Model file for the job. Use its own axes, mm. A direction names the side the tool comes from. Round coordinates to 2 decimals unless told otherwise and drop trailing zeros. Order: outer loops, then holes, each group sorted by start corner. A loop starts at its lowest first (then second) coordinate and runs counter-clockwise, first axis right, second up. Notation, with made-up numbers: (-29.5, 17.5) - (23.5, 17.5) arc R25 ccw to (23.5, 52.5) - close; hole circle Ø5 at (5.25, -7). An arc over 180 degrees is marked (long way). Put each result on its own line as item: value. Start each with the question number.
Item 1: Probe probe 1 along Y at (x, z) = (2.5, 1.35); probe 2 along Y at (x, z) = (5.75, 0.8); probe 3 along X at (y, z) = (1, 0.8). List the from-to ranges inside material, lowest first.
Item 2: Saw through at A-A on x = 6.75. List the corners of the cut face in (y, z), plus the area to 3 significant figures.
Item 3: Which spindle directions (+Z, -Z, +X, -X, +Y, -Y) get a long thin tool onto all of the face, cutting with end or side? Do faces 4 (the face through (0.89, 2.04, 0)), 5 (the face through (-0.822, -3, 1)). Say none if no direction does.
Item 4: Saw through at B-B on y = 10.5. List the corners of the cut face in (x, z).
Item 5: Saw through at C-C on z = 1.15. List the corners of the cut face in (x, y).
Item 6: Saw through at D-D on x = 5.25. State how many separate pieces and enclosed holes the cut face has, plus the area to 3 significant figures.
Item 7: Mould opens along Y. For faces 1 (the face through (3.7, -14.195, 1.1)), 2 (the face through (3, -15.195, 1)), 3 (the face through (-1, 2, 1.4)) say: pulls with the +Y half, pulls with the -Y half, needs draft (parallel to the pull), parting line crosses it, or undercut.
```python
from build123d import *

# Parameters (mm, degrees)
SKETCH_1_W           = 10
SKETCH_1_H           = 34
EXTRUDE_2_DEPTH      = 1.4
SKETCH_2_W           = 8
SKETCH_2_H           = 32
CUT_EXTRUDE_1_DEPTH  = 1.2
SKETCH_4_W           = 1.2
SKETCH_4_H           = 1
CUT_EXTRUDE_4_DEPTH  = 1.2
FILLET_1_R           = 0.5
FILLET_2_R           = 0.5
SKETCH_6_W           = 6.011424245
SKETCH_6_H           = 0.514664245
CUT_EXTRUDE_6_DEPTH  = 0.5
SKETCH_7_W           = 0.498386998
SKETCH_7_H           = 14.972688723
CUT_EXTRUDE_7_DEPTH  = 0.5
SKETCH_8_W           = 0.497690278
SKETCH_8_H           = 27.903913782
CUT_EXTRUDE_8_DEPTH  = 0.5
SKETCH_10_W          = 5.67106867
SKETCH_10_H          = 0.515598409
CUT_EXTRUDE_9_DEPTH  = 0.5
CUT_EXTRUDE_11_REACH = 22.554


with BuildPart() as part:
    # 草图1 → 凸台-拉伸2 (new body)
    with BuildSketch(Plane.XY):
        with Locations((3.178294574, 1.80536099)):
            Rectangle(SKETCH_1_W, SKETCH_1_H)
    extrude(amount=EXTRUDE_2_DEPTH)

    # 草图2 → 切除-拉伸1 (cut)
    with BuildSketch(Plane.XY.offset(1.4)):
        with Locations((3.178294574, 1.80536099)):
            Rectangle(SKETCH_2_W, SKETCH_2_H)
    extrude(amount=-CUT_EXTRUDE_1_DEPTH, mode=Mode.SUBTRACT)

    # 草图4 → 切除-拉伸4 (cut)
    with BuildSketch(Plane.XY.offset(1.4)):
        with Locations((-0.221705426, -14.69463901)):
            Rectangle(SKETCH_4_W, SKETCH_4_H)
    extrude(amount=-CUT_EXTRUDE_4_DEPTH, mode=Mode.SUBTRACT)

    # 圆角1
    fillet_1_edges = [part.edges().sort_by_distance(p)[0] for p in [
        (-1.821705426, -15.19463901, 0.7),
    ]]
    fillet(fillet_1_edges, radius=FILLET_1_R)

    # 圆角2
    fillet_2_edges = [part.edges().sort_by_distance(p)[0] for p in [
        (-1.821705426, 18.80536099, 0.7),
        (8.178294574, 18.80536099, 0.7),
        (8.178294574, -15.19463901, 0.7),
    ]]
    fillet(fillet_2_edges, radius=FILLET_2_R)

    # 草图6 → 切除-拉伸6 (cut)
    with BuildSketch(Plane.XZ.offset(-17.80536099)):
        with Locations((3.184006697, 0.642667877)):
            Rectangle(SKETCH_6_W, SKETCH_6_H)
    extrude(amount=-CUT_EXTRUDE_6_DEPTH, mode=Mode.SUBTRACT)

    # 草图7 → 切除-拉伸7 (cut)
    with BuildSketch(Plane(origin=(-0.821705426, 0, 0), x_dir=(0, 0, -1), z_dir=(1, 0, 0))):
        with Locations((-0.650806501, 8.293480481)):
            Rectangle(SKETCH_7_W, SKETCH_7_H)
    extrude(amount=-CUT_EXTRUDE_7_DEPTH, mode=Mode.SUBTRACT)

    # 草图8 → 切除-拉伸8 (cut)
    with BuildSketch(Plane.ZY.offset(-7.178294574)):
        with Locations((0.641533001, 1.822842427)):
            Rectangle(SKETCH_8_W, SKETCH_8_H)
    extrude(amount=-CUT_EXTRUDE_8_DEPTH, mode=Mode.SUBTRACT)

    # 草图10 → 切除-拉伸9 (cut)
    with BuildSketch(Plane(origin=(0, -14.19463901, 0), x_dir=(1, 0, 0), z_dir=(0, 1, 0))):
        with Locations((3.213828909, -0.642200795)):
            Rectangle(SKETCH_10_W, SKETCH_10_H)
    extrude(amount=-CUT_EXTRUDE_9_DEPTH, mode=Mode.SUBTRACT)

    # 草图11 → 切除-拉伸11 (cut, up to next)
    with BuildSketch(Plane(origin=(0, 0, 0), x_dir=(-1, 0, 0), z_dir=(0, 0, -1)), mode=Mode.PRIVATE) as cut_extrude_11_sk1:
        with BuildLine():
            Line((-4.31947378, 17.019101686), (-0.131341084, 13.086732818))
            ThreePointArc((-0.131341084, 13.086732818), (-0.078041772, 11.394479644), (-1.770294947, 11.341180331))
            Line((-1.770294947, 11.341180331), (-5.958427643, 15.273549198))
            ThreePointArc((-5.958427643, 15.273549198), (-6.011726955, 16.965802373), (-4.31947378, 17.019101686))
        make_face()
    cut_extrude_11_tool1 = extrude(cut_extrude_11_sk1.sketch, amount=-CUT_EXTRUDE_11_REACH, mode=Mode.PRIVATE) & part.part
    # 草图11 → 切除-拉伸11 (cut, up to next)
    with BuildSketch(Plane(origin=(0, 0, 0), x_dir=(-1, 0, 0), z_dir=(0, 0, -1)), mode=Mode.PRIVATE) as cut_extrude_11_sk2:
        with BuildLine():
            Line((-5.958427643, 9.273549198), (-1.770294947, 5.341180331))
            ThreePointArc((-1.770294947, 5.341180331), (-0.078041772, 5.394479644), (-0.131341084, 7.086732818))
            Line((-0.131341084, 7.086732818), (-4.31947378, 11.019101686))
            ThreePointArc((-4.31947378, 11.019101686), (-6.011726955, 10.965802373), (-5.958427643, 9.273549198))
        make_face()
    cut_extrude_11_tool2 = extrude(cut_extrude_11_sk2.sketch, amount=-CUT_EXTRUDE_11_REACH, mode=Mode.PRIVATE) & part.part
    # 草图11 → 切除-拉伸11 (cut, up to next)
    with BuildSketch(Plane(origin=(0, 0, 0), x_dir=(-1, 0, 0), z_dir=(0, 0, -1)), mode=Mode.PRIVATE) as cut_extrude_11_sk3:
        with BuildLine():
            Line((-5.958427643, 3.273549198), (-1.770294947, -0.658819669))
            ThreePointArc((-1.770294947, -0.658819669), (-0.078041772, -0.605520356), (-0.131341084, 1.086732818))
            Line((-0.131341084, 1.086732818), (-4.31947378, 5.019101686))
            ThreePointArc((-4.31947378, 5.019101686), (-6.011726955, 4.965802373), (-5.958427643, 3.273549198))
        make_face()
    cut_extrude_11_tool3 = extrude(cut_extrude_11_sk3.sketch, amount=-CUT_EXTRUDE_11_REACH, mode=Mode.PRIVATE) & part.part
    # 草图11 → 切除-拉伸11 (cut, up to next)
    with BuildSketch(Plane(origin=(0, 0, 0), x_dir=(-1, 0, 0), z_dir=(0, 0, -1)), mode=Mode.PRIVATE) as cut_extrude_11_sk4:
        with BuildLine():
            Line((-5.958427643, -2.726450802), (-1.770294947, -6.658819669))
            ThreePointArc((-1.770294947, -6.658819669), (-0.078041772, -6.605520356), (-0.131341084, -4.913267182))
            Line((-0.131341084, -4.913267182), (-4.31947378, -0.980898314))
            ThreePointArc((-4.31947378, -0.980898314), (-6.011726955, -1.034197627), (-5.958427643, -2.726450802))
        make_face()
    cut_extrude_11_tool4 = extrude(cut_extrude_11_sk4.sketch, amount=-CUT_EXTRUDE_11_REACH, mode=Mode.PRIVATE) & part.part
    # 草图11 → 切除-拉伸11 (cut, up to next)
    with BuildSketch(Plane(origin=(0, 0, 0), x_dir=(-1, 0, 0), z_dir=(0, 0, -1)), mode=Mode.PRIVATE) as cut_extrude_11_sk5:
        with BuildLine():
            Line((-5.958427643, -8.726450802), (-1.770294947, -12.658819669))
            ThreePointArc((-1.770294947, -12.658819669), (-0.078041772, -12.605520356), (-0.131341084, -10.913267182))
            Line((-0.131341084, -10.913267182), (-4.31947378, -6.980898314))
            ThreePointArc((-4.31947378, -6.980898314), (-6.011726955, -7.034197627), (-5.958427643, -8.726450802))
        make_face()
    cut_extrude_11_tool5 = extrude(cut_extrude_11_sk5.sketch, amount=-CUT_EXTRUDE_11_REACH, mode=Mode.PRIVATE) & part.part
    add(cut_extrude_11_tool1.solids().sort_by_distance((3.044884, 14.180141, 0))[0], mode=Mode.SUBTRACT)
    add(cut_extrude_11_tool2.solids().sort_by_distance((3.044884, 8.180141, 0))[0], mode=Mode.SUBTRACT)
    add(cut_extrude_11_tool3.solids().sort_by_distance((3.044884, 2.180141, 0))[0], mode=Mode.SUBTRACT)
    add(cut_extrude_11_tool4.solids().sort_by_distance((3.044884, -3.819859, 0))[0], mode=Mode.SUBTRACT)
    add(cut_extrude_11_tool5.solids().sort_by_distance((3.044884, -9.819859, 0))[0], mode=Mode.SUBTRACT)


solid = part.part
```
Results found:
1. probe 1: y = -15.19 to -14.19, 17.81 to 18.81
1. probe 2: y = -15.19 to -14.69, 18.31 to 18.81
1. probe 3: x = -1.82 to -1.32, 7.68 to 8.18
2. outline: (-15.19, 0) - (18.81, 0) - (18.81, 1.4) - (17.81, 1.4) - (17.81, 0.2) - (-14.19, 0.2) - (-14.19, 1.4) - (-15.19, 1.4) - close
2. area: 9.20 mm²
3. face 4: -Z, +X, -X, +Y, -Y
3. face 5: +Z, -Y
4. outline: (-1.82, 0) - (3.77, 0) - (3.77, 0.2) - (-0.82, 0.2) - (-0.82, 0.4) - (-1.32, 0.4) - (-1.32, 0.9) - (-0.82, 0.9) - (-0.82, 1.4) - (-1.82, 1.4) - close; (6.28, 0) - (8.18, 0) - (8.18, 1.4) - (7.18, 1.4) - (7.18, 0.89) - (7.68, 0.89) - (7.68, 0.39) - (7.18, 0.39) - (7.18, 0.2) - (6.28, 0.2) - close
5. outline: (-1.82, -14.69) arc R0.5 ccw to (-1.32, -15.19) - (-0.82, -15.19) - (-0.82, 17.81) - (7.18, 17.81) - (7.18, -14.19) - (0.38, -14.19) - (0.38, -15.19) - (7.68, -15.19) arc R0.5 ccw to (8.18, -14.69) - (8.18, 18.31) arc R0.5 ccw to (7.68, 18.81) - (-1.32, 18.81) arc R0.5 ccw to (-1.82, 18.31) - close
6. separate pieces: 6
6. enclosed holes: 0
6. area: 5.95 mm²
7. face 1: undercut
7. face 2: pulls with the -Y half
7. face 3: needs draft
